```python
from build123d import *

# Parameters (mm, degrees)
SKETCH2_W           = 330.2
SKETCH2_H           = 19.05
BOSS_EXTRUDE1_DEPTH = 63.5
SKETCH4_R           = 4.699
CUT_EXTRUDE2_DEPTH  = 20.05


with BuildPart() as part:
    # Sketch2 → Boss-Extrude1 (new body)
    with BuildSketch(Plane.XY):
        with Locations((0, 9.525)):
            Rectangle(SKETCH2_W, SKETCH2_H)
    extrude(amount=BOSS_EXTRUDE1_DEPTH)

    # Sketch4 → Cut-Extrude2 (cut, through all)
    with BuildSketch(Plane(origin=(0, 0, 0), x_dir=(1, 0, 0), z_dir=(0, 1, 0))):
        with Locations((0, -31.75)):
            Circle(SKETCH4_R)
    extrude(amount=CUT_EXTRUDE2_DEPTH, mode=Mode.SUBTRACT)


solid = part.part
```
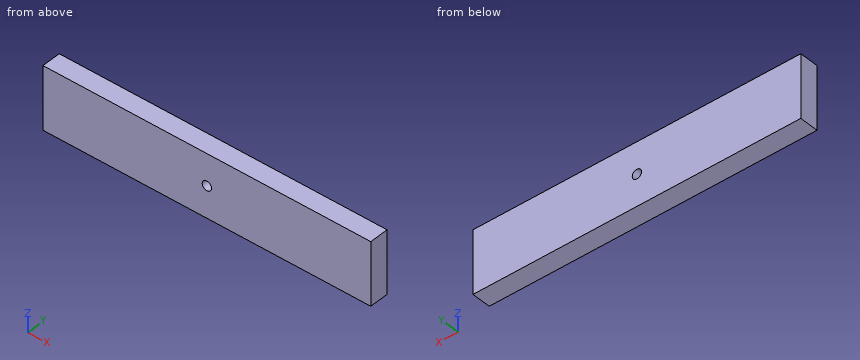
Could you check a few things on this model? Use its own coordinates, in mm. Coordinates: 2 decimals unless noted, no trailing zeros. Write each loop counter-clockwise with the first axis right and the second up, starting at its lowest first coordinate (ties: lowest second). Pieces come first, ordered by that corner, then holes. Notation, with made-up numbers: (35.25, 13) -> (94.25, 13) arc R29 cw to (94.25, 39) -> close; hole circle Ø3 at (-11, -32.5). An arc over 180 degrees is marked (long way). Write item = value, one per line. Start each with the question number.
(1) I need wall thicknesses on line 1 (X direction, y = 13.5, z = 31.75); line 2 (Z direction, x = 0, y = 8.5); line 3 (X direction, y = 9, z = 34.5). Which ranges of each line are inside material? Lowest first, please. Write a range as [from, to].
(2) I want a section at B-B (z = 31.75). Please give me the cut outline in (x, y).
(3) I want a section at A-A (x = 0). Please give me the cut outline in (y, z), plus the area to 3 significant figures.
Result set:
q1.line_1 = [-165.1, -4.7], [4.7, 165.1]
q1.line_2 = [0, 27.05], [36.45, 63.5]
q1.line_3 = [-165.1, -3.81], [3.81, 165.1]
q2.outline = (-165.1, 0) -> (-4.7, 0) -> (-4.7, 19.05) -> (-165.1, 19.05) -> close; (4.7, 0) -> (165.1, 0) -> (165.1, 19.05) -> (4.7, 19.05) -> close
q3.outline = (0, 0) -> (19.05, 0) -> (19.05, 27.05) -> (0, 27.05) -> close; (0, 36.45) -> (19.05, 36.45) -> (19.05, 63.5) -> (0, 63.5) -> close
q3.area = 1,030 mm2
